Could you check a few things on this drawing? It's one solid part, dimensions in mm from its lowest x, y, z. Coordinates: 2 decimals unless noted, no trailing zeros. Loops run counter-clockwise (first coordinate to the right, second up) from the corner with the lowest first, then second, coordinate; pieces in that order, holes last. Notation, with made-up numbers: (70, 58) -> (80, 58) arc R12 ccw to (80, 73) -> close; hole circle Ø3 at (6.5, -26). An arc over 180 degrees is marked (long way). One line per question, with ' | ' between items. Start each with the question number.
(1) If we mould it in two halves opening along Z, with no side actions, what happens to the marked faces 1 and 2? For each: pulls with the +Z half, pulls with the -Z half, needs draft (parallel to the pull), parting line crosses it, or undercut.
(2) Suppose I cut it at C-C (y = 91). Please give me the cut outline in (x, z), plus the area to 3 significant figures.
(3) Suppose I cut it at B-B (y = 67.5). Please give me the cut outline in (x, z), plus the area to 3 significant figures.
(4) I'm going to push flat-ended pins straight in: pin 1 Ø1.5 at (y, z) = (36.5, 12) entering from +X (1 decimal); pin 2 Ø5 at (y, z) = (45.5, 11.5) entering from -X; pin 3 Ø6 at (x, y) = (11.5, 11) entering from -Z. Where does each tip first touch, or does it pass through?
(5) Suppose I cut it at A-A (z = 13.5). Please give me the cut outline in (x, y).
(6) Suppose I cut it at D-D (x = 13). Please give me the cut outline in (y, z).
(7) If I drill on line 1 along X through (y, z) = (89.75, 7.5); line 2 along X through (y, z) = (31.5, 5); line 3 along X through (y, z) = (24, 11.5) (1 decimal), over which ranges is the centre line in solid material (lowest first)?
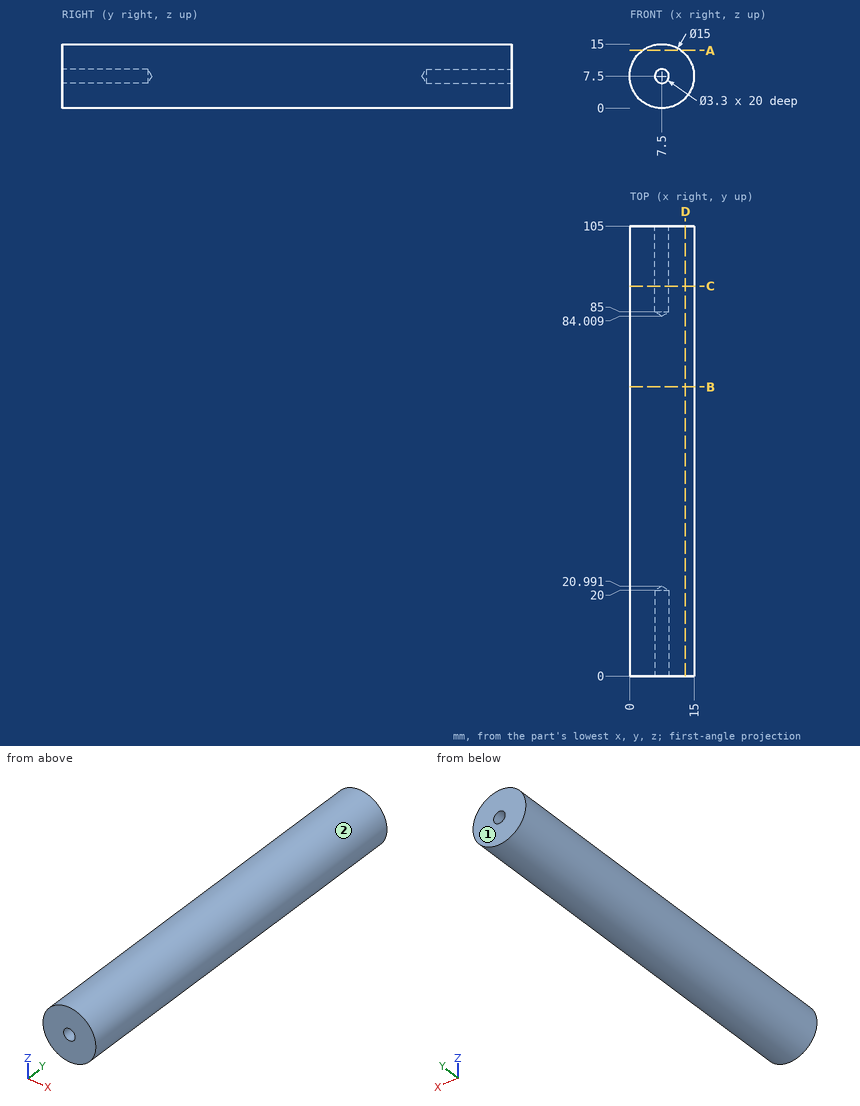
Checks:
1) face 1: needs draft | face 2: parting line crosses it
2) outline: circle Ø15 at (7.5, 7.5); hole circle Ø3.3 at (7.5, 7.5) | area: 168 mm^2
3) outline: circle Ø15 at (7.5, 7.5) | area: 177 mm^2
4) pin 1: stops at x = 14 | pin 2: stops at x = 0.15 | pin 3: stops at z = 0.07
5) outline: (3, 0) -> (12, 0) -> (12, 105) -> (3, 105) -> close
6) outline: (0, 2.4) -> (105, 2.4) -> (105, 12.6) -> (0, 12.6) -> close
7) line 1: x = 0 to 5.85, 9.15 to 15 | line 2: x = 0.43 to 14.57 | line 3: x = 1.2 to 13.8
